Verification items for the finished model (mm, model axes). A direction names the side the tool comes from. Give positions to 0.01 mm unless a question says otherwise; leave off trailing zeros. Loops run counter-clockwise (first coordinate to the right, second up) from the corner with the lowest first, then second, coordinate; pieces in that order, holes last. Notation, with made-up numbers: (66, -29) - (117, -29) arc R21 ccw to (117, -18) - close; hole circle Ø10 at (-16, -2). An arc over 180 degrees is marked (long way). One line per question, with ' | ' between items. Start each with the question number.
1. Tool access check on faces 1 (the face through (-7.493, -4.437, -0.33)), 2 (the face through (-2, 5, -6)). Record the directions out of +Z, -Z, +X, -X, +Y, -Y that give a thin tool (end or side, any length) a straight path to the whole face; none if there is none.
2. Section check D-D, the plane y = -4.5. Enter the section's corners in (x, z), then the cut area to 3 significant figures.
3. Depth check by flat-ended pin: pin 1 Ø6 at (y, z) = (5.5, 5.5) entering from -X; pin 2 Ø1.5 at (x, y) = (1, 6) entering from +Z. Enter the tip coordinate at first touch or a pass-through.
4. Section check B-B, the plane x = -0.75. Enter the section's corners in (y, z), then the cut area to 3 significant figures.
5. Section check C-C, the plane y = 9. Enter the section's corners in (x, z).
6. Section check A-A, the plane z = 0. Enter the section's corners in (x, y), then the cut area to 3 significant figures.
7. Thickness scan on line 1 along Z through (x, y) = (0, 19); line 2 along X through (y, z) = (10, -0.5); line 3 along Z through (x, y) = (-3.25, -4.5). Record the ranges inside material, lowest first. Write a range as from..to.
Autodesk Inventor part; units mm, degrees
ref_plane "Work Plane1" through (0, 12.5, 0) normal (0, 1, 0) x (1, 0, 0)
ref_plane "YZ Plane" through (0, 0, 0) normal (1, 0, 0) x (0, 1, 0)
ref_plane "XZ Plane" through (0, 0, 0) normal (0, 1, 0) x (-1, 0, 0)
sketch "Sketch1" plane through (0, 0, 0) normal (0, 1, 0) x (-1, 0, 0)
  circle A0 centre (0, 0) radius 6.5
  dimension "d0" = 13
extrude "Extrusion1" add sketch "Sketch1" along normal blind 5
sketch "Sketch2" plane through (0, 0, 0) normal (0, -1, 0) x (1, 0, 0)
  circle A0 centre (0, 0) radius 7.5
  dimension "d3" = 15
extrude "Extrusion2" add sketch "Sketch2" along normal blind 9
sketch "Sketch3" plane through (0, 5, 0) normal (0, 1, 0) x (1, 0, 0)
  circle A0 centre (0, 0) radius 6
  dimension "d6" = 12
extrude "Extrusion3" add sketch "Sketch3" along normal blind 19
ref_plane "Work Plane1" through (0, 12.5, 0) normal (0, 1, 0) x (1, 0, 0)
sketch "Sketch4" plane through (0, 12.5, 0) normal (0, 1, 0) x (1, 0, 0)
  circle A0 centre (0, 0) radius 6
  circle A1 centre (0, 0) radius 6
properties part number "plunger" material "ABS Plastic"
Results list:
1) face 1: +Y, -Y | face 2: +Y
2) outline: circle Ø15 at (0, 0) | area: 177 mm²
3) pin 1: x = -5.98 | pin 2: z = 5.99
4) outline: (-9, -7.46) - (0, -7.46) - (0, -6.46) - (5, -6.46) - (5, -5.95) - (24, -5.95) - (24, 5.95) - (5, 5.95) - (5, 6.46) - (0, 6.46) - (0, 7.46) - (-9, 7.46) - close | area: 425 mm²
5) outline: circle Ø12 at (0, 0)
6) outline: (-7.5, -9) - (7.5, -9) - (7.5, 0) - (6.5, 0) - (6.5, 5) - (6, 5) - (6, 24) - (-6, 24) - (-6, 5) - (-6.5, 5) - (-6.5, 0) - (-7.5, 0) - close | area: 428 mm²
7) line 1: -6..6 | line 2: -5.98..5.98 | line 3: -6.76..6.76
